from build123d import *

# Parameters (mm, degrees)
SKETCH1_W           = 38.1
SKETCH1_H           = 25.4
BOSS_EXTRUDE1_DEPTH = 19.05
SKETCH2_R           = 1.5875
CUT_EXTRUDE2_DEPTH  = 25.4
SKETCH3_W           = 12.108446299
SKETCH3_H           = 19.05
CUT_EXTRUDE3_DEPTH  = 19.05
SKETCH4_W           = 19.05
SKETCH4_H           = 12.7
CUT_EXTRUDE4_DEPTH  = 50.8
SKETCH6_W           = 7.660570014
SKETCH6_H           = 3.81
BOSS_EXTRUDE2_DEPTH = 7.62
CUT_EXTRUDE6_DEPTH  = 19.05
SKETCH8_W           = 5.08
SKETCH8_H           = 2.54
BOSS_EXTRUDE3_DEPTH = 2.54
SKETCH9_R           = 0.508
CUT_EXTRUDE7_DEPTH  = 19.05
SKETCH10_W          = 9.525
SKETCH10_H          = 19.05
CUT_EXTRUDE8_DEPTH  = 3.81


with BuildPart() as part:
    # Sketch1 → Boss-Extrude1 (new body)
    with BuildSketch(Plane(origin=(0, 0, 0), x_dir=(1, 0, 0), z_dir=(0, 1, 0))):
        with Locations((-3.175, 0)):
            Rectangle(SKETCH1_W, SKETCH1_H)
    extrude(amount=BOSS_EXTRUDE1_DEPTH)

    # Sketch2 → Cut-Extrude2 (cut)
    with BuildSketch(Plane.XY.offset(12.7)):
        with Locations((-12.7, 9.525)):
            Circle(SKETCH2_R)
        with BuildLine():
            ThreePointArc((-12.7, 19.05), (-22.225, 9.525), (-12.7, 0))
            ThreePointArc((-12.7, 0), (-33.665146333, 9.525), (-12.7, 19.05))
        make_face()
        with BuildLine():
            ThreePointArc((6.35, 0), (15.875, 9.525), (6.35, 19.05))
            ThreePointArc((6.35, 19.05), (24.948138119, 9.525), (6.35, 0))
        make_face()
    extrude(amount=-CUT_EXTRUDE2_DEPTH, mode=Mode.SUBTRACT)

    # Sketch3 → Cut-Extrude3 (cut)
    with BuildSketch(Plane(origin=(0, 19.05, 0), x_dir=(1, 0, 0), z_dir=(0, 1, 0))):
        with Locations((-18.754223149, 0)):
            Rectangle(SKETCH3_W, SKETCH3_H)
    extrude(amount=-CUT_EXTRUDE3_DEPTH, mode=Mode.SUBTRACT)

    # Sketch4 → Cut-Extrude4 (cut)
    with BuildSketch(Plane(origin=(-15.875, 0, 0), x_dir=(0, 0, -1), z_dir=(1, 0, 0))):
        with Locations((0, 9.525)):
            Rectangle(SKETCH4_W, SKETCH4_H)
    extrude(amount=CUT_EXTRUDE4_DEPTH, mode=Mode.SUBTRACT)

    # Sketch6 → Boss-Extrude2 (add)
    with BuildSketch(Plane(origin=(0, 0, 0), x_dir=(1, 0, 0), z_dir=(0, 1, 0))):
        with Locations((-2.519714993, 0)):
            Rectangle(SKETCH6_W, SKETCH6_H)
    extrude(amount=-BOSS_EXTRUDE2_DEPTH)

    # Sketch7 → Cut-Extrude6 (cut)
    with BuildSketch(Plane.XY.offset(12.7)):
        with BuildLine():
            Line((-7.080935196, -3.131729905), (-6.858, 0))
            Line((-6.858, 0), (-6.858, -7.767816491))
            Line((-6.858, -7.767816491), (-14.771031914, -7.767816491))
            Line((-14.771031914, -7.767816491), (-14.771031914, 0))
            Line((-14.771031914, 0), (-9.975013633, 0))
            ThreePointArc((-9.975013633, 0), (-9.162678538, -1.206904896), (-8.794375076, -2.614335284))
            ThreePointArc((-8.794375076, -2.614335284), (-9.25025826, -3.647474967), (-10.163496252, -4.311706442))
            ThreePointArc((-10.163496252, -4.311706442), (-11.221462334, -3.861030674), (-11.89339597, -2.927807191))
            ThreePointArc((-11.89339597, -2.927807191), (-11.604147707, -2.390005207), (-10.996168015, -2.332941862))
            ThreePointArc((-10.996168015, -2.332941862), (-10.54556137, -1.577353268), (-11.301149964, -1.126746624))
            ThreePointArc((-11.301149964, -1.126746624), (-12.52752029, -1.573373178), (-13.044460874, -2.771802103))
            ThreePointArc((-13.044460874, -2.771802103), (-12.016160281, -5.071387383), (-9.595781192, -5.769427237))
            ThreePointArc((-9.595781192, -5.769427237), (-7.890109837, -4.877949662), (-7.080935196, -3.131729905))
        make_face()
        with BuildLine():
            Line((1.563031914, 0), (-3.232986367, 0))
            ThreePointArc((-3.232986367, 0), (-4.045321462, -1.206904896), (-4.413624924, -2.614335284))
            ThreePointArc((-4.413624924, -2.614335284), (-3.95774174, -3.647474967), (-3.044503748, -4.311706442))
            ThreePointArc((-3.044503748, -4.311706442), (-1.986537666, -3.861030674), (-1.31460403, -2.927807191))
            ThreePointArc((-1.31460403, -2.927807191), (-1.603852293, -2.390005207), (-2.211831985, -2.332941862))
            ThreePointArc((-2.211831985, -2.332941862), (-2.66243863, -1.577353268), (-1.906850036, -1.126746624))
            ThreePointArc((-1.906850036, -1.126746624), (-0.68047971, -1.573373178), (-0.163539126, -2.771802103))
            ThreePointArc((-0.163539126, -2.771802103), (-1.191839719, -5.071387383), (-3.612218808, -5.769427237))
            ThreePointArc((-3.612218808, -5.769427237), (-5.317890163, -4.877949662), (-6.127064804, -3.131729905))
            Line((-6.127064804, -3.131729905), (-6.35, 0))
            Line((-6.35, 0), (-6.35, -7.767816491))
            Line((-6.35, -7.767816491), (1.563031914, -7.767816491))
            Line((1.563031914, -7.767816491), (1.563031914, 0))
        make_face()
    extrude(amount=-CUT_EXTRUDE6_DEPTH, mode=Mode.SUBTRACT)

    # Sketch8 → Boss-Extrude3 (add)
    with BuildSketch(Plane(origin=(0, 19.05, 0), x_dir=(1, 0, 0), z_dir=(0, 1, 0))):
        Rectangle(SKETCH8_W, SKETCH8_H)
    extrude(amount=BOSS_EXTRUDE3_DEPTH)

    # Sketch9 → Cut-Extrude7 (cut)
    with BuildSketch(Plane.XY.offset(12.7)):
        with Locations((0, 20.32)):
            Circle(SKETCH9_R)
        with BuildLine():
            ThreePointArc((-2.54, 19.05), (0, 21.59), (2.54, 19.05))
            ThreePointArc((2.54, 19.05), (0, 23.383223271), (-2.54, 19.05))
        make_face()
    extrude(amount=-CUT_EXTRUDE7_DEPTH, mode=Mode.SUBTRACT)

    # Sketch10 → Cut-Extrude8 (cut)
    with BuildSketch(Plane(origin=(0, 19.05, 0), x_dir=(1, 0, 0), z_dir=(0, 1, 0))):
        with Locations((-7.9375, 0)):
            Rectangle(SKETCH10_W, SKETCH10_H)
    extrude(amount=-CUT_EXTRUDE8_DEPTH, mode=Mode.SUBTRACT)


solid = part.part
The model under review builds one solid part; all positions refer to its coordinate system, in mm. A direction names the side the tool comes from. Coordinates: 2 decimals unless noted, no trailing zeros. Order: outer loops, then holes, each group sorted by start corner. A loop starts at its lowest first (then second) coordinate and runs counter-clockwise, first axis right, second up. Notation, with made-up numbers: (43.25, 10.25) -> (58.25, 10.25) arc R18 cw to (58.25, 26.25) -> close; hole circle Ø6 at (71.25, 76). An arc over 180 degrees is marked (long way). Answer in a Markdown table with one row per item.
(1) Consider section D-D (z = -5). Write out the cut boundary in (x, y) (3 decimals), plus the area to 3 significant figures.
Answers:
| item | result |
|---|---|
| outline | (-12.7, 0) -> (6.35, 0) arc R9.525 ccw to (13.45, 3.175) -> (-12.7, 3.175) -> close; (-3.175, 15.875) -> (13.45, 15.875) arc R9.525 ccw to (6.35, 19.05) -> (-3.175, 19.05) -> close |
| area | 122 mm² |
(2) The part is to be moulded in two halves that separate along Z. For faces 1 (the flat face through (-5, -3, 1.905)), 2 (the flat face through (-3, 10, -9.525)), 3 (the cylindrical face through (-1.596, -2.395, 0.027)), say which applies: +Z half, -Z half, draft (parallel to the pull), parting line (faces both ways), or undercut.
Answers:
| item | result |
|---|---|
| face 1 | +Z half |
| face 2 | undercut |
| face 3 | draft |
(3) Insertion check: pin 1 (8.5 mm diameter, centred on x = 5.5, z = 0.5, fed in from -Y); pin 2 (10 mm diameter, centred on y = 4, z = 7, fed in from +X); pin 3 (2 mm diameter, centred on x = 8.5, z = -3.5, fed in from -Y). Each pin has a flat end and moves straight along its axis. Give the tip position at first contact, or say it passes through.
Answers:
| item | result |
|---|---|
| pin 1 | y = 0 |
| pin 2 | x = 15.8 |
| pin 3 | y = 0.07 |
(4) Consider section A-A (x = 3.5). Write out the cut boundary in (y, z) (3 decimals), plus the area to 3 significant figures.
Answers:
| item | result |
|---|---|
| outline | (0, -12.7) -> (19.05, -12.7) -> (19.05, 12.7) -> (0, 12.7) -> close; hole (3.175, -9.525) -> (15.875, -9.525) -> (15.875, 9.525) -> (3.175, 9.525) -> close |
| area | 242 mm² |
(5) Machinability: for faces 4 (the flat face through (0, 3.175, 0)), 5 (the flat face through (1, 20, -1.27)), 6 (the cylindrical face through (-4.037, -1.188, 0.027)), 7 (the flat face through (-12.7, 2, 0)), which of the approach directions +Z, -Z, +X, -X, +Y, -Y give a long, thin tool a straight path to every point of the face, cutting with its end or side? Answer none if there is none.
Answers:
| item | result |
|---|---|
| face 4 | +X, -X |
| face 5 | -Z, +X, -X, +Y |
| face 6 | +Z, -Z |
| face 7 | -X, +Y, -Y |
(6) Wall thickness on line 1 along Y through (x, z) = (-12.7, 11.8); line 2 along Z through (x, y) = (13, 4) (3 decimals): over which ranges is each line inside the solid? List them lowest first.
Answers:
| item | result |
|---|---|
| line 1 | 0 to 7.94, 11.11 to 19.05 |
| line 2 | -12.7 to -9.525, 9.525 to 12.7 |
(7) Consider section B-B (z = -0.5). State how many separate pieces and enclosed holes the cut face has, plus the area to 3 significant figures.
Answers:
| item | result |
|---|---|
| separate pieces | 2 |
| enclosed holes | 1 |
| area | 151 mm² |
(8) Consider section C-C (x = -13.5). Write out the cut boundary in (y, z) (3 decimals), plus the area to 3 significant figures.
Answers:
| item | result |
|---|---|
| outline | (0.034, -12.7) -> (8.154, -12.7) -> (8.154, -9.525) -> (0.034, -9.525) -> close; (0.034, 9.525) -> (8.154, 9.525) -> (8.154, 12.7) -> (0.034, 12.7) -> close; (10.896, -12.7) -> (19.016, -12.7) -> (19.016, -9.525) -> (10.896, -9.525) -> close; (10.896, 9.525) -> (19.016, 9.525) -> (19.016, 12.7) -> (10.896, 12.7) -> close |
| area | 103 mm² |
